The figure shows three views and two pictorial views of one solid part (mm, origin at its lowest corner). Answer the questions. Coordinates: 2 decimals unless noted, no trailing zeros. Loops run counter-clockwise (first coordinate to the right, second up) from the corner with the lowest first, then second, coordinate; pieces in that order, holes last.
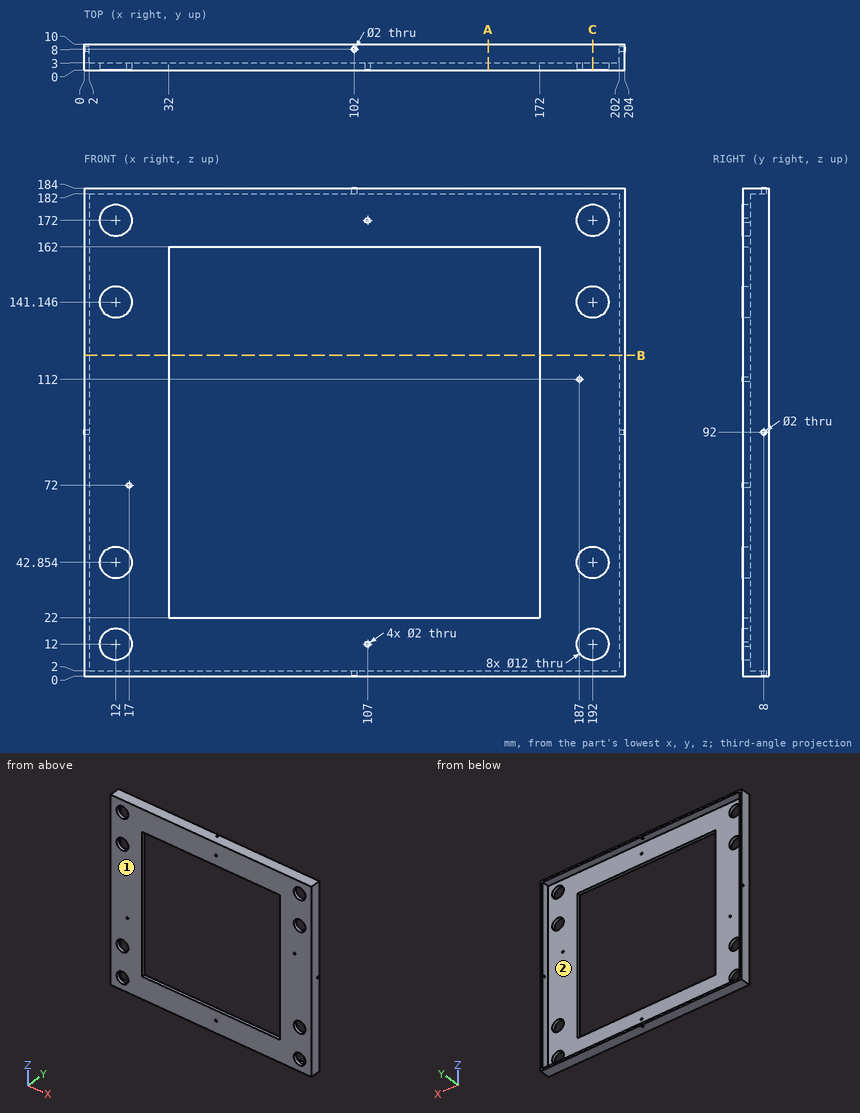
Q1. A cutting plane is placed at A-A (x = 152.5). Give the vertices of the cut face in (y, z), then the cut area to 3 significant figures.
Findings below:
outline: (0, 0) - (10, 0) - (10, 2) - (3, 2) - (3, 22) - (0, 22) - close; (0, 162) - (3, 162) - (3, 182) - (10, 182) - (10, 184) - (0, 184) - close
area: 160 mm2
Q2. Straight lines are drawn through the part: probe 1 along X at (y, z) = (1.35, 172); probe 2 along X at (y, z) = (3.5, 153.5); probe 3 along Y at (x, z) = (202.5, 92). For each, find the intervals that lie inside material, in ascending order.
Findings below:
probe 1: x = 0 to 6, 18 to 106, 108 to 186, 198 to 204
probe 2: x = 0 to 2, 202 to 204
probe 3: y = 0 to 7, 9 to 10
Q3. A cutting plane is placed at B-B (z = 121). Give the vertices of the cut face in (x, y).
Findings below:
outline: (0, 0) - (32, 0) - (32, 3) - (2, 3) - (2, 10) - (0, 10) - close; (172, 0) - (204, 0) - (204, 10) - (202, 10) - (202, 3) - (172, 3) - close
Q4. A cutting plane is placed at C-C (x = 192). Give the vertices of the cut face in (y, z).
Findings below:
outline: (0, 0) - (10, 0) - (10, 2) - (3, 2) - (3, 6) - (0, 6) - close; (0, 18) - (3, 18) - (3, 36.85) - (0, 36.85) - close; (0, 48.85) - (3, 48.85) - (3, 135.15) - (0, 135.15) - close; (0, 147.15) - (3, 147.15) - (3, 166) - (0, 166) - close; (0, 178) - (3, 178) - (3, 182) - (10, 182) - (10, 184) - (0, 184) - close
Q5. Flat-ended cylindrical pins translate along their axes: pin 1 Ø3.5 at (x, y) = (96, 1.5) entering from -Z; pin 2 Ø19 at (x, z) = (12, 42.85) entering from +Y. Find the tip coordinate at first contact, or state that the pin passes through.
Findings below:
pin 1: stops at z = 0
pin 2: stops at y = 3
Q6. Determine the mould class of the marked faces 1 and 2 for opening direction Z: +Z half, -Z half, draft (parallel to the pull), parting line (faces both ways), or undercut.
Findings below:
face 1: draft
face 2: undercut
